from build123d import *

# Parameters (mm, degrees)
SKETCH2_W          = 9.186415934
SKETCH2_H          = 0.97118121
SKETCH2_W_2        = 0.97118121
SKETCH2_H_2        = 9.186415934
CUT_EXTRUDE1_DEPTH = 1.27


with BuildPart() as part:
    # Sketch1 → Revolve1 (revolve)
    with BuildSketch(Plane(origin=(0, 0, 0), x_dir=(1, 0, 0), z_dir=(0, 1, 0))):
        with BuildLine():
            Line((0, 47.625), (0, 0))
            Line((0, 0), (0, -3.175))
            Line((0, -3.175), (1.5875, -3.175))
            ThreePointArc((1.5875, -3.175), (4.429777637, -2.770069708), (7.045889178, -1.5875))
            Line((7.045889178, -1.5875), (7.045889178, 0))
            Line((7.045889178, 0), (3.175, 0))
            Line((3.175, 0), (3.175, 47.625))
            Line((3.175, 47.625), (7.045889178, 47.625))
            Line((7.045889178, 47.625), (7.045889178, 49.2125))
            ThreePointArc((7.045889178, 49.2125), (4.429777637, 50.395069708), (1.5875, 50.8))
            Line((1.5875, 50.8), (0, 50.8))
            Line((0, 50.8), (0, 47.625))
        make_face()
    revolve(axis=Axis((0, 0, 0), (0, 0, -1)))

    # Sketch2 → Cut-Extrude1 (cut)
    with BuildSketch(Plane.XY.offset(3.175)):
        Rectangle(SKETCH2_W, SKETCH2_H)
        Rectangle(SKETCH2_W_2, SKETCH2_H_2)
    cut_extrude1 = extrude(amount=-CUT_EXTRUDE1_DEPTH, mode=Mode.SUBTRACT)

    # Mirror1: Cut-Extrude1 across plane
    add(cut_extrude1.mirror(Plane(origin=(0, 0, -23.8125), x_dir=(1, 0, 0), z_dir=(0, 0, -1))), mode=Mode.SUBTRACT)


solid = part.part
Geometry: final body of the model. Coordinates: model frame, mm. A direction names the side the tool comes from. Give positions to 0.01 mm unless a question says otherwise; leave off trailing zeros. Write each loop counter-clockwise with the first axis right and the second up, starting at its lowest first coordinate (ties: lowest second). Pieces come first, ordered by that corner, then holes.
(1) Ray query, line 1 (Z direction, x = 4, y = -1.75) (3 decimals); line 2 (Z direction, x = 3.25, y = -1.5) (3 decimals); line 3 (Y direction, x = -0.25, z = -43). Return the intervals inside material, ascending.
(2) First-contact query: P1, Ø1, axis at y = 2.5, z = 2.5, coming from the -X side; P2, Ø0.6, axis at x = -2.5, z = -50, coming from the -Y side; P3, Ø8, axis at y = -3, z = -24, coming from the +X side (3 decimals); P4, Ø1.5, axis at x = -5, z = -42.5, coming from the +Y side (3 decimals). Flat tips, straight axial feed; report the tip coordinate or a pass-through.
(3) Cut plane A-A, the plane z = -31. Return loops of the section in (x, y) (3 decimals).
(4) Access query for faces 1 (the flat face through (-0.486, 2.5, 2.5)), 2 (the flat face through (-3, -0.486, -50)), 3 (the flat face through (1, 1, 3.175)). Directions: +Z, -Z, +X, -X, +Y, -Y. A direction counts if a zero-diameter tool reaches every point of the face in a straight line with its end or side. Return the directions, or none.
(5) Mould query, pull axis X, two halves, no side actions, for faces 4 (the flat face through (-3, 1.5, -47.625)), 5 (the cylindrical face through (-7.04, -0.31, 0.78)), 6 (the flat face through (-2.6, -0.486, 2.5)). Classes: released by +X, released by -X, zero draft, split by the parting line, or undercut.
Values follow:
1. line 1: z = -50.413 to -47.625, 0 to 2.788
1. line 2: z = -50.603 to -47.625, 0 to 2.978
1. line 3: y = -3.17 to 3.17
2. P1: stops at x = -5.84
2. P2: stops at y = -5.68
2. P3: stops at x = 3.175
2. P4: passes through
3. outline: circle Ø6.35 at (0, 0)
4. face 1: +Z
4. face 2: -Z
4. face 3: +Z, +X, -X, +Y, -Y
5. face 4: zero draft
5. face 5: split by the parting line
5. face 6: undercut
